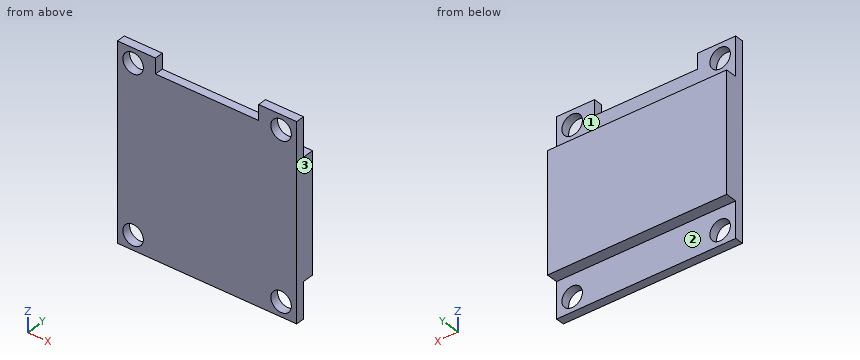
from build123d import *

# Parameters (mm, degrees)
SKETCH1_W           = 25
SKETCH1_H           = 27
BOSS_EXTRUDE1_DEPTH = 1.2
SKETCH2_W           = 25
SKETCH2_H           = 16.6
BOSS_EXTRUDE2_DEPTH = 1.6
SKETCH3_R           = 1.43
SKETCH3_W           = 14.4
SKETCH3_H           = 2.13
CUT_EXTRUDE1_DEPTH  = 1.2


with BuildPart() as part:
    # Sketch1 → Boss-Extrude1 (new body)
    with BuildSketch(Plane(origin=(0, 0, 0), x_dir=(1, 0, 0), z_dir=(0, 1, 0))):
        Rectangle(SKETCH1_W, SKETCH1_H)
    extrude(amount=BOSS_EXTRUDE1_DEPTH)

    # Sketch2 → Boss-Extrude2 (add)
    with BuildSketch(Plane(origin=(0, 1.2, 0), x_dir=(1, 0, 0), z_dir=(0, 1, 0))):
        with Locations((0, 0.2)):
            Rectangle(SKETCH2_W, SKETCH2_H)
    extrude(amount=BOSS_EXTRUDE2_DEPTH)

    # Sketch3 → Cut-Extrude1 (cut)
    with BuildSketch(Plane(origin=(0, 1.2, 0), x_dir=(1, 0, 0), z_dir=(0, 1, 0))):
        with Locations(Location((10.32, 11.47, 0), (0, 0, 270))):
            Circle(SKETCH3_R)
        with Locations(Location((-10.32, 11.47, 0), (0, 0, 270))):
            Circle(SKETCH3_R)
        with Locations(Location((-10.32, -11.47, 0), (0, 0, 270))):
            Circle(SKETCH3_R)
        with Locations(Location((10.32, -11.47, 0), (0, 0, 270))):
            Circle(SKETCH3_R)
        with Locations((0, -12.435)):
            Rectangle(SKETCH3_W, SKETCH3_H)
    extrude(amount=-CUT_EXTRUDE1_DEPTH, mode=Mode.SUBTRACT)


solid = part.part
Geometry check sheet. Reference: the model listing, model coordinates, mm. Face numbers are marked on the shaded views. A direction names the side the tool comes from. Give positions to 0.01 mm unless a question says otherwise; leave off trailing zeros. Loops run counter-clockwise (first coordinate to the right, second up) from the corner with the lowest first, then second, coordinate; pieces in that order, holes last. Notation, with made-up numbers: M 81.5,73.25 L 124.5,73.25 A14 cw 124.5,99.25 Z; hole C 13.5,12 d1. An arc over 180 degrees is marked long. Write each question's results on one line, items separated by ' | '.
1) Section check A-A, the plane z = -11.47. Record the boundary of the cut face in (x, y), plus the area to 3 significant figures.
Answers follow:
outline: M -12.5,0 L -11.75,0 L -11.75,1.2 L -12.5,1.2 Z; M -8.89,0 L 8.89,0 L 8.89,1.2 L -8.89,1.2 Z; M 11.75,0 L 12.5,0 L 12.5,1.2 L 11.75,1.2 Z | area: 23.1 mm2
2) Tool access check on the marked faces 1, 2 and 3. Record the directions out of +Z, -Z, +X, -X, +Y, -Y that give a thin tool (end or side, any length) a straight path to the whole face; none if there is none.
Answers follow:
face 1: +Z, +X, -X, +Y | face 2: -Z, +X, -X, +Y | face 3: +Z, -Z, +X, +Y, -Y
3) Section check B-B, the plane y = 0.75. Record the boundary of the cut face in (x, z), plus the area to 3 significant figures.
Answers follow:
outline: M -12.5,-13.5 L 12.5,-13.5 L 12.5,13.5 L 7.2,13.5 L 7.2,11.37 L -7.2,11.37 L -7.2,13.5 L -12.5,13.5 Z; hole C -10.32,-11.47 d2.86; hole C -10.32,11.47 d2.86; hole C 10.32,-11.47 d2.86; hole C 10.32,11.47 d2.86 | area: 619 mm2
4) Section check C-C, the plane x = -10.32. Record the boundary of the cut face in (y, z).
Answers follow:
outline: M 0,-13.5 L 1.2,-13.5 L 1.2,-12.9 L 0,-12.9 Z; M 0,-10.04 L 1.2,-10.04 L 1.2,-8.5 L 2.8,-8.5 L 2.8,8.1 L 1.2,8.1 L 1.2,10.04 L 0,10.04 Z; M 0,12.9 L 1.2,12.9 L 1.2,13.5 L 0,13.5 Z
5) Gauge pin test, flat ends, axial feed: pin 1 (3.5 mm diameter, centred on x = -10.32, z = 11.47, fed in from +Y); pin 2 (2.5 mm diameter, centred on x = 10.32, z = -11.47, fed in from +Y) (3 decimals); pin 3 (0.5 mm diameter, centred on x = 2.5, y = 2, fed in from +Z); pin 4 (1.3 mm diameter, centred on x = 6, y = 2, fed in from -Z). Record the tip position at first contact, or that the pin passes through.
Answers follow:
pin 1: y = 1.2 | pin 2: through | pin 3: z = 8.1 | pin 4: z = -8.5
6) Thickness scan on line 1 (X direction, y = 0.8, z = 11.47); line 2 (X direction, y = 1, z = -11.47); line 3 (Z direction, x = 8.5, y = 2.6). Record the ranges inside material, lowest first.
Answers follow:
line 1: -12.5 to -11.75, -8.89 to -7.2, 7.2 to 8.89, 11.75 to 12.5 | line 2: -12.5 to -11.75, -8.89 to 8.89, 11.75 to 12.5 | line 3: -8.5 to 8.1
7) Section check D-D, the plane x = 6. Record the boundary of the cut face in (y, z).
Answers follow:
outline: M 0,-13.5 L 1.2,-13.5 L 1.2,-8.5 L 2.8,-8.5 L 2.8,8.1 L 1.2,8.1 L 1.2,11.37 L 0,11.37 Z
